Part model, mm, in its own coordinate system. Round coordinates to 2 decimals unless told otherwise and drop trailing zeros. Loops run counter-clockwise (first coordinate to the right, second up) from the corner with the lowest first, then second, coordinate; pieces in that order, holes last. Notation, with made-up numbers: M 87,19 L 142,19 A35 ccw 142,55 Z; hole C -13.5,-10.75 d2. An arc over 180 degrees is marked long. Write each question's results on one line, items separated by ' | '.
from build123d import *

# Parameters (mm, degrees)
BOSS_EXTRUDE1_DEPTH      = 1.5
BOSS_EXTRUDE1_DEPTH_BACK = 1.5
CUT_EXTRUDE1_DEPTH       = 106.28456677


with BuildPart() as part:
    # Sketch1 → Boss-Extrude1 (new, two sides: drawn at the far end of the back side and taken through both)
    with BuildSketch(Plane(origin=(0, 0, 0), x_dir=(0, 0, -1), z_dir=(1, 0, 0)).offset(-BOSS_EXTRUDE1_DEPTH_BACK)):
        with BuildLine():
            Line((-80, 30), (-87, 30))
            Line((-87, 30), (-87, 32.6))
            Line((-87, 32.6), (-93, 32.6))
            Line((-93, 32.6), (-93, 30))
            Line((-93, 30), (-100, 30))
            ThreePointArc((-100, 30), (-96.828033965, 18.713629613), (-99.446714265, 7.28620477))
            ThreePointArc((-99.446714265, 7.28620477), (-98.266775294, 1.214741861), (-92.088027506, 0.935468515))
            ThreePointArc((-92.088027506, 0.935468515), (-67.824329395, 9.838481267), (-42.435753596, 5))
            ThreePointArc((-42.435753596, 5), (-32.005584176, 1.266555107), (-21, 0))
            Line((-21, 0), (-18, 0))
            Line((-18, 0), (-18, 2.8))
            Line((-18, 2.8), (-14, 2.8))
            Line((-14, 2.8), (-14, 0))
            Line((-14, 0), (-10.5, 0))
            Line((-10.5, 0), (-10.5, 2.8))
            Line((-10.5, 2.8), (-2.5, 2.8))
            Line((-2.5, 2.8), (-2.5, 10.133333333))
            Line((-2.5, 10.133333333), (-5.5, 10.133333333))
            Line((-5.5, 10.133333333), (-5.5, 12.733333333))
            Line((-5.5, 12.733333333), (-2.5, 12.733333333))
            Line((-2.5, 12.733333333), (-2.5, 20.066666667))
            Line((-2.5, 20.066666667), (-5.5, 20.066666667))
            Line((-5.5, 20.066666667), (-5.5, 22.666666667))
            Line((-5.5, 22.666666667), (-2.5, 22.666666667))
            Line((-2.5, 22.666666667), (-2.5, 30))
            Line((-2.5, 30), (-10.5, 30))
            Line((-10.5, 30), (-10.5, 32.8))
            Line((-10.5, 32.8), (-14, 32.8))
            Line((-14, 32.8), (-14, 30))
            Line((-14, 30), (-17.249742261, 30))
            ThreePointArc((-17.249742261, 30), (-22.023510763, 15.292477496), (-37.40016873, 13.661994841))
            ThreePointArc((-37.40016873, 13.661994841), (-57.183488606, 19.61610248), (-77.802405966, 18.315567968))
            ThreePointArc((-77.802405966, 18.315567968), (-81.536934186, 19.325375212), (-82.669963788, 23.024382595))
            ThreePointArc((-82.669963788, 23.024382595), (-81.611172702, 26.61790516), (-80, 30))
        make_face()
    extrude(amount=BOSS_EXTRUDE1_DEPTH + BOSS_EXTRUDE1_DEPTH_BACK)

    # Sketch2 → Cut-Extrude1 (cut, through all)
    with BuildSketch(Plane(origin=(1.5, 0, 0), x_dir=(0, 0, -1), z_dir=(1, 0, 0))):
        Polygon((-7.833333333, 30), (-5.166666667, 30), (-2.5, 30), (-2.5, 29), (-7.833333333, 29), align=None)
    extrude(amount=-CUT_EXTRUDE1_DEPTH, mode=Mode.SUBTRACT)


solid = part.part
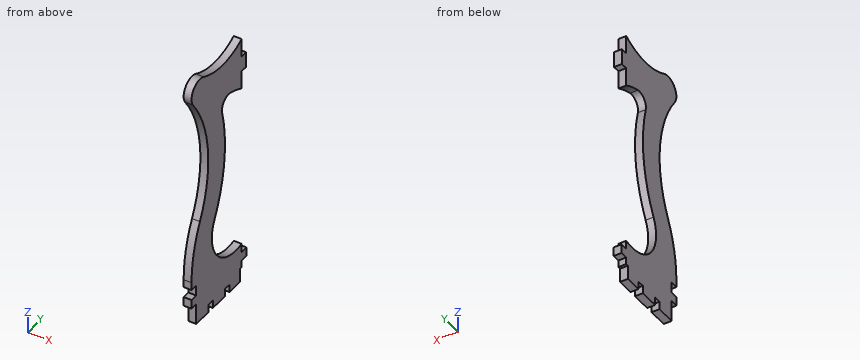
Item 1: Band-saw the part on C-C on z = 58.5. Give the cut face in (x, y).
Filled sheet:
outline: M -1.5,9.7 L 1.5,9.7 L 1.5,19.75 L -1.5,19.75 Z
Item 2: Wall check: L1, parallel to Z at x = -1, y = 30.5; L2, parallel to Z at x = -1.2, y = 22.5; L3, parallel to Y at x = -0.35, z = 42. Give the ranges that are in metal, low to high.
Filled sheet:
L1: 10.5 to 14, 87 to 93 | L2: 5.5 to 17.29, 82.74 to 97.23 | L3: 4.79 to 15.75
Item 3: Drop flat-ended pins along their axis: P1, Ø1.5, axis at x = -0.5, z = 97, coming from the +Y side; P2, Ø0.9, axis at x = 0, z = 4, coming from the -Y side; P3, Ø8, axis at y = 5.5, z = 65.5, coming from the +X side; P4, Ø1.4, axis at x = -0.5, y = 1, coming from the +Z side. Give the stop position or say it passes through.
Filled sheet:
P1: y = 30 | P2: y = 2.8 | P3: through | P4: z = 98.76
Item 4: Band-saw the part on A-A on y = 24. Give the cut face in (x, z).
Filled sheet:
outline: M -1.5,2.5 L 1.5,2.5 L 1.5,16.96 L -1.5,16.96 Z; M -1.5,82.44 L 1.5,82.44 L 1.5,97.56 L -1.5,97.56 Z
Item 5: Band-saw the part on B-B on y = 14.5. Give the cut face in (x, z), and give its area (3 significant figures).
Filled sheet:
outline: M -1.5,2.5 L 1.5,2.5 L 1.5,23.1 L -1.5,23.1 Z; M -1.5,39.12 L 1.5,39.12 L 1.5,97.1 L -1.5,97.1 Z | area: 236 mm^2
Item 6: Band-saw the part on D-D on z = 31.5. Give the cut face in (x, y).
Filled sheet:
outline: M -1.5,1.15 L 1.5,1.15 L 1.5,12.13 L -1.5,12.13 Z
